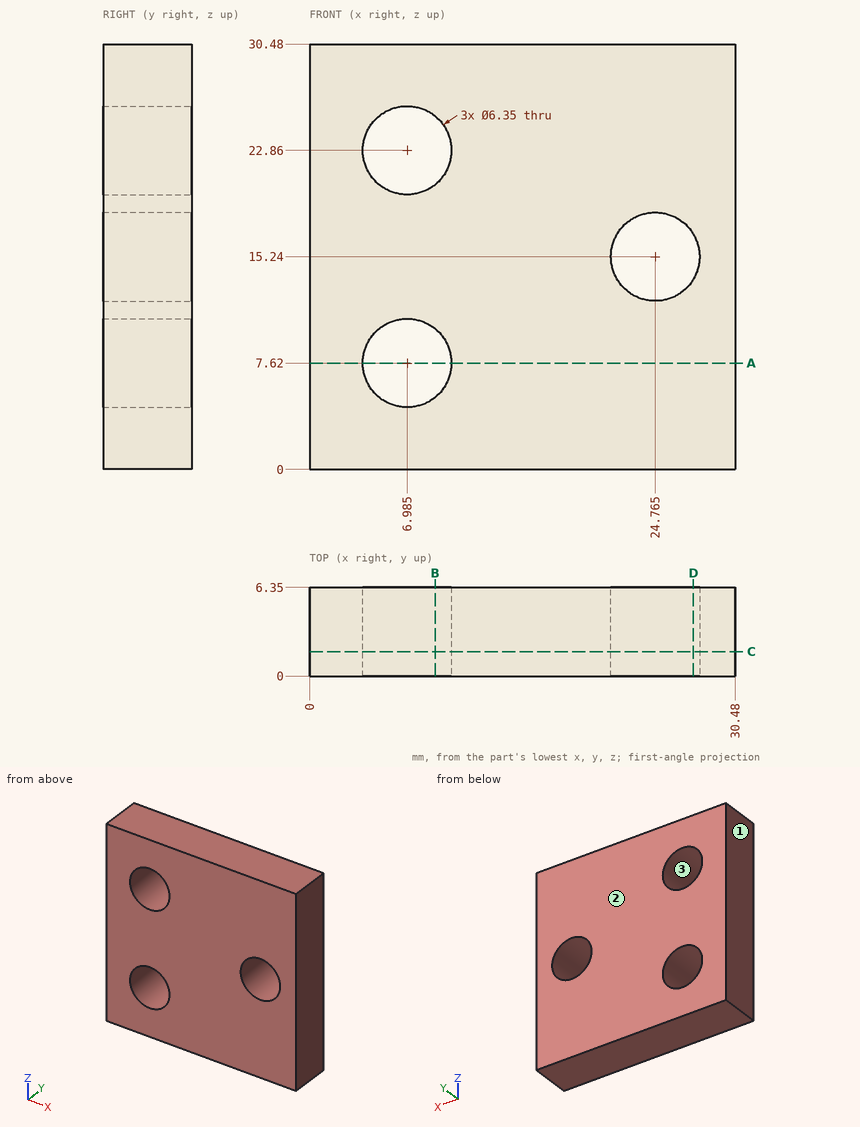
Source: three-view drawing plus pictorial views. Frame: mm from the lowest corner of the part. Round coordinates to 2 decimals unless told otherwise and drop trailing zeros. Loops run counter-clockwise (first coordinate to the right, second up) from the corner with the lowest first, then second, coordinate; pieces in that order, holes last.
1. Section query A-A on z = 7.62. Output: boundary loops of the cut face in (x, y).
2. Ray query, L1, parallel to Z at x = 7, y = 1.5; L2, parallel to X at y = 2.5, z = 15.24; L3, parallel to X at y = 3.75, z = 22.86. Return the intervals inside material, ascending.
3. Section query D-D on x = 27.5. Output: boundary loops of the cut face in (y, z), and give its area (3 significant figures).
4. Section query B-B on x = 9. Output: boundary loops of the cut face in (y, z).
5. Mould query, pull axis X, two halves, no side actions, for the marked faces 1, 2 and 3. Classes: released by +X, released by -X, zero draft, split by the parting line, or undercut.
6. Section query C-C on y = 1.75. Output: boundary loops of the cut face in (x, z) (3 decimals), and give its area (3 significant figures).
Answers below:
1. outline: (0, 0) - (3.81, 0) - (3.81, 6.35) - (0, 6.35) - close; (10.16, 0) - (30.48, 0) - (30.48, 6.35) - (10.16, 6.35) - close
2. L1: z = 0 to 4.45, 10.79 to 19.69, 26.03 to 30.48
2. L2: x = 0 to 21.59, 27.94 to 30.48
2. L3: x = 0 to 3.81, 10.16 to 30.48
3. outline: (0, 0) - (6.35, 0) - (6.35, 13.63) - (0, 13.63) - close; (0, 16.85) - (6.35, 16.85) - (6.35, 30.48) - (0, 30.48) - close
3. area: 173 mm2
4. outline: (0, 0) - (6.35, 0) - (6.35, 5.17) - (0, 5.17) - close; (0, 10.07) - (6.35, 10.07) - (6.35, 20.41) - (0, 20.41) - close; (0, 25.31) - (6.35, 25.31) - (6.35, 30.48) - (0, 30.48) - close
5. face 1: released by -X
5. face 2: zero draft
5. face 3: undercut
6. outline: (0, 0) - (30.48, 0) - (30.48, 30.48) - (0, 30.48) - close; hole circle Ø6.35 at (6.985, 7.62); hole circle Ø6.35 at (6.985, 22.86); hole circle Ø6.35 at (24.765, 15.24)
6. area: 834 mm2
